```python
from build123d import *

# Parameters (mm, degrees)
SKETCH1_W           = 127
SKETCH1_H           = 101.6
BOSS_EXTRUDE1_DEPTH = 2.54
SKETCH2_W           = 127
SKETCH2_H           = 101.6
SKETCH2_W_2         = 121.92
SKETCH2_H_2         = 96.52
BOSS_EXTRUDE2_DEPTH = 22.86
FILLET1_R           = 10.16
FILLET2_R           = 12.7
SKETCH3_R           = 1.016
CUT_EXTRUDE1_DEPTH  = 2.54
SKETCH4_W           = 10.922
SKETCH4_H           = 5.08
CUT_EXTRUDE2_DEPTH  = 2.54
FILLET3_R           = 1.27
SKETCH6_R           = 0.635
CUT_EXTRUDE4_DEPTH  = 7.62


with BuildPart() as part:
    # Sketch1 → Boss-Extrude1 (new body)
    with BuildSketch(Plane(origin=(0, 0, 0), x_dir=(1, 0, 0), z_dir=(0, 1, 0))):
        with Locations((63.5, 50.8)):
            Rectangle(SKETCH1_W, SKETCH1_H)
    extrude(amount=BOSS_EXTRUDE1_DEPTH)

    # Sketch2 → Boss-Extrude2 (add)
    with BuildSketch(Plane(origin=(0, 2.54, 0), x_dir=(1, 0, 0), z_dir=(0, 1, 0))):
        with Locations((63.5, 50.8)):
            Rectangle(SKETCH2_W, SKETCH2_H)
        with Locations((63.5, 50.8)):
            Rectangle(SKETCH2_W_2, SKETCH2_H_2, mode=Mode.SUBTRACT)
    extrude(amount=BOSS_EXTRUDE2_DEPTH)

    # Fillet1
    fillet1_edges = [part.edges().sort_by_distance(p)[0] for p in [
        (124.46, 13.97, -99.06),
        (2.54, 13.97, -99.06),
        (2.54, 13.97, -2.54),
        (124.46, 13.97, -2.54),
    ]]
    fillet(fillet1_edges, radius=FILLET1_R)

    # Fillet2
    fillet2_edges = [part.edges().sort_by_distance(p)[0] for p in [
        (0, 12.7, -101.6),
        (127, 12.7, -101.6),
        (127, 12.7, 0),
        (0, 12.7, 0),
    ]]
    fillet(fillet2_edges, radius=FILLET2_R)

    # Sketch3 → Cut-Extrude1 (cut)
    with BuildSketch(Plane(origin=(127, 0, 0), x_dir=(0, 0, -1), z_dir=(1, 0, 0))):
        with Locations((50.8, 12.7)):
            Circle(SKETCH3_R)
        with Locations((58.42, 12.7)):
            Circle(SKETCH3_R)
        with Locations((66.04, 12.7)):
            Circle(SKETCH3_R)
        with Locations((73.66, 12.7)):
            Circle(SKETCH3_R)
        with Locations((81.28, 12.7)):
            Circle(SKETCH3_R)
        with Locations((43.18, 12.7)):
            Circle(SKETCH3_R)
        with Locations((35.56, 12.7)):
            Circle(SKETCH3_R)
        with Locations((27.94, 12.7)):
            Circle(SKETCH3_R)
        with Locations((20.32, 12.7)):
            Circle(SKETCH3_R)
        with Locations((20.32, 19.05)):
            Circle(SKETCH3_R)
        with Locations((27.94, 19.05)):
            Circle(SKETCH3_R)
        with Locations((35.56, 19.05)):
            Circle(SKETCH3_R)
        with Locations((43.18, 19.05)):
            Circle(SKETCH3_R)
        with Locations((50.8, 19.05)):
            Circle(SKETCH3_R)
        with Locations((58.42, 19.05)):
            Circle(SKETCH3_R)
        with Locations((66.04, 19.05)):
            Circle(SKETCH3_R)
        with Locations((73.66, 19.05)):
            Circle(SKETCH3_R)
        with Locations((81.28, 19.05)):
            Circle(SKETCH3_R)
        with Locations((20.32, 6.35)):
            Circle(SKETCH3_R)
        with Locations((27.94, 6.35)):
            Circle(SKETCH3_R)
        with Locations((35.56, 6.35)):
            Circle(SKETCH3_R)
        with Locations((43.18, 6.35)):
            Circle(SKETCH3_R)
        with Locations((50.8, 6.35)):
            Circle(SKETCH3_R)
        with Locations((58.42, 6.35)):
            Circle(SKETCH3_R)
        with Locations((66.04, 6.35)):
            Circle(SKETCH3_R)
        with Locations((73.66, 6.35)):
            Circle(SKETCH3_R)
        with Locations((81.28, 6.35)):
            Circle(SKETCH3_R)
    extrude(amount=-CUT_EXTRUDE1_DEPTH, mode=Mode.SUBTRACT)

    # Sketch4 → Cut-Extrude2 (cut)
    with BuildSketch(Plane.ZY):
        with Locations((-82.677, 5.842)):
            Rectangle(SKETCH4_W, SKETCH4_H)
    extrude(amount=-CUT_EXTRUDE2_DEPTH, mode=Mode.SUBTRACT)

    # Fillet3
    fillet3_edges = [part.edges().sort_by_distance(p)[0] for p in [
        (1.27, 8.382, -77.216),
        (1.27, 8.382, -88.138),
        (1.27, 3.302, -88.138),
        (1.27, 3.302, -77.216),
    ]]
    fillet(fillet3_edges, radius=FILLET3_R)

    # Sketch6 → Cut-Extrude4 (cut)
    with BuildSketch(Plane(origin=(0, 25.4, 0), x_dir=(1, 0, 0), z_dir=(0, 1, 0))):
        with Locations(Location((4.681771045, 4.708740144, 0), (0, 0, 270))):
            Circle(SKETCH6_R)
        with Locations(Location((4.681771045, 96.891259856, 0), (0, 0, 270))):
            Circle(SKETCH6_R)
        with Locations(Location((122.318228955, 96.891259856, 0), (0, 0, 270))):
            Circle(SKETCH6_R)
        with Locations(Location((122.318228955, 4.708740144, 0), (0, 0, 270))):
            Circle(SKETCH6_R)
    extrude(amount=-CUT_EXTRUDE4_DEPTH, mode=Mode.SUBTRACT)


solid = part.part
```
The model under review builds one solid part; all positions refer to its coordinate system, in mm. A direction names the side the tool comes from. Give positions to 0.01 mm unless a question says otherwise; leave off trailing zeros. Write each loop counter-clockwise with the first axis right and the second up, starting at its lowest first coordinate (ties: lowest second). Pieces come first, ordered by that corner, then holes. Notation, with made-up numbers: M -36.5,26 L -25.5,26 A6 ccw -25.5,36 Z; hole C 37.25,69 d5. An arc over 180 degrees is marked long. Answer in a Markdown table with one row per item.
Item 1: For line 1 along Y through (x, z) = (125.2, -81.28); line 2 along X through (y, z) = (21, -81); line 3 along Z through (x, y) = (50.5, 23), list the stretches that pass through material, from the lowest coordinate up.
Check sheet entries:
| item | result |
|---|---|
| line 1 | 0 to 5.33, 7.37 to 11.68, 13.72 to 18.03, 20.07 to 25.4 |
| line 2 | 0 to 2.54, 124.46 to 127 |
| line 3 | -101.6 to -99.06, -2.54 to 0 |
Item 2: For P1, Ø1, axis at x = 122, z = -5, coming from the +Y side; P2, Ø0.8, axis at x = 4.68, z = -96.89, coming from the +Y side; P3, Ø5, axis at x = 32, z = -90.5, coming from the +Y side; P4, Ø1.8, axis at y = 12.7, z = -73.66, coming from the +X side, all flat-tipped, find the tip position at first contact; note any pin that passes through.
Check sheet entries:
| item | result |
|---|---|
| P1 | y = 25.4 |
| P2 | y = 17.78 |
| P3 | y = 2.54 |
| P4 | x = 2.54 |
Item 3: Add section A-A on y = 16. Give the boundary of the cut face in (x, z).
Check sheet entries:
| item | result |
|---|---|
| outline | M 0,-88.9 A12.7 ccw 12.7,-101.6 L 114.3,-101.6 A12.7 ccw 127,-88.9 L 127,-12.7 A12.7 ccw 114.3,0 L 12.7,0 A12.7 ccw 0,-12.7 Z; hole M 2.54,-88.9 A10.16 ccw 12.7,-99.06 L 114.3,-99.06 A10.16 ccw 124.46,-88.9 L 124.46,-12.7 A10.16 ccw 114.3,-2.54 L 12.7,-2.54 A10.16 ccw 2.54,-12.7 Z |
Item 4: Draft analysis for pull direction X (two halves, no side actions). For faces 1 (the face through (121.563, 14.13, -5.595)), 2 (the face through (5.437, 14.13, -96.005)), 3 (the face through (1, 6, -77.216)), 4 (the face through (3.62, 12.52, -97.78)), state which applies: +X half, -X half, draft (parallel to the pull), parting line (faces both ways), or undercut.
Check sheet entries:
| item | result |
|---|---|
| face 1 | undercut |
| face 2 | undercut |
| face 3 | draft |
| face 4 | -X half |
Item 5: Add section B-B on x = 87.5. Give the boundary of the cut face in (y, z), plus the area to 3 significant figures.
Check sheet entries:
| item | result |
|---|---|
| outline | M 0,-101.6 L 25.4,-101.6 L 25.4,-99.06 L 2.54,-99.06 L 2.54,-2.54 L 25.4,-2.54 L 25.4,0 L 0,0 Z |
| area | 374 mm2 |
Item 6: Tool access review of faces 5 (the face through (1, 3.302, -83)), 6 (the face through (3.62, 12.88, -3.82)), 7 (the face through (63, 2.54, -51)): name each direction out of +Z, -Z, +X, -X, +Y, -Y from which nothing blocks a thin tool from reaching the whole face with its end or side.
Check sheet entries:
| item | result |
|---|---|
| face 5 | -X |
| face 6 | +Z, -X, +Y, -Y |
| face 7 | +Y |
